Autodesk Inventor part; units mm, degrees
ref_plane "YZ Plane" through (0, 0, 0) normal (1, 0, 0) x (0, 1, 0)
ref_plane "XZ Plane" through (0, 0, 0) normal (0, 1, 0) x (-1, 0, 0)
ref_plane "XY Plane" through (0, 0, 0) normal (0, 0, 1) x (1, 0, 0)
sketch "Skizze1" plane through (0, 0, 0) normal (0, 0, 1) x (1, 0, 0)
  line L0 (-4.75, 4.75) -> (4.75, 4.75)
  line L1 (4.75, 4.75) -> (4.75, -4.75)
  line L2 (4.75, -4.75) -> (-4.75, -4.75)
  line L3 (-4.75, -4.75) -> (-4.75, 4.75)
  line L4 (-4.75, 4.75) -> (4.75, -4.75) construction
  line L5 (4.75, 4.75) -> (-4.75, -4.75) construction
  point P0 (0, 0)
  dimension "d0" = 9.5
  dimension "d1" = 9.5
extrude "Extrusion1" add sketch "Skizze1" along normal blind 3.5
sketch "Skizze2" plane through (0, 0, 3.5) normal (0, 0, 1) x (1, 0, 0)
  circle A0 centre (0, 0) radius 8.5
  dimension "d4" = 17
extrude "Extrusion2" add sketch "Skizze2" along normal blind 3
sketch "Skizze3" plane through (0, 0, 6.5) normal (0, 0, 1) x (1, 0, 0)
  circle A0 centre (0, 0) radius 7.4
  circle A1 centre (0, 0) radius 8.5
  dimension "d7" = 14.8
  dimension "d19" = 1.1
extrude "Extrusion3" add sketch "Skizze3" along normal blind 96 contours A0
sketch "Skizze4" plane through (0, 0, 102.5) normal (0, 0, 1) x (1, 0, 0)
  line L0 (-4.75, -4.75) -> (4.75, -4.75)
  line L1 (-4.75, 4.75) -> (4.75, 4.75)
  line L2 (4.75, 4.75) -> (4.75, -4.75)
  line L3 (4.75, -4.75) -> (-4.75, -4.75)
  line L4 (-4.75, -4.75) -> (-4.75, 4.75)
  line L5 (-4.75, 4.75) -> (4.75, -4.75) construction
  line L6 (4.75, 4.75) -> (-4.75, -4.75) construction
  point P0 (0, 0)
  dimension "d10" = 9.5
extrude "Extrusion4" add sketch "Skizze4" along normal blind 6
sketch "Skizze5" plane through (0, 0, 108.5) normal (0, 0, 1) x (1, 0, 0)
  circle A0 centre (0, 0) radius 2.25
  dimension "d13" = 4.5
extrude "Extrusion5" cut sketch "Skizze5" against normal blind 5
sketch "Skizze6" plane through (0, 0, 0) normal (0, 0, -1) x (-1, 0, 0)
  circle A0 centre (0, 0) radius 2.25
  dimension "d16" = 4.5
extrude "Extrusion6" cut sketch "Skizze6" against normal blind 5
properties part number "_3D-Druck"
Work out the finished part from the listing and answer in its coordinate system (mm). A direction names the side the tool comes from. Give positions to 0.01 mm unless a question says otherwise; leave off trailing zeros. Write each loop counter-clockwise with the first axis right and the second up, starting at its lowest first coordinate (ties: lowest second). Pieces come first, ordered by that corner, then holes.
(1) Flat-ended cylindrical pins translate along their axes: pin 1 Ø4 at (y, z) = (1.5, 2) entering from -X; pin 2 Ø1 at (x, y) = (1.5, 6) entering from -Z; pin 3 Ø3 at (x, z) = (2.5, 2.5) entering from -Y. Find the tip coordinate at first contact, or state that the pin passes through.
Final values:
pin 1: stops at x = -8.5
pin 2: stops at z = 3.5
pin 3: stops at y = -8.39
(2) The mould has two halves that part along X. Classify faces 5 (the cylindrical face through (0.29, 2.23, 2.46)), 6 (the flat face through (0, -6, 3.5)), 7 (the flat face through (4.75, 0, 2)): pulls with the +X half, pulls with the -X half, needs draft (parallel to the pull), parting line crosses it, or undercut.
Final values:
face 5: undercut
face 6: needs draft
face 7: pulls with the +X half
(3) The part is cut by section D-D on y = -6. Write down the section's boundary in (x, z).
Final values:
outline: (-6.02, 3.5) - (6.02, 3.5) - (6.02, 6.5) - (4.33, 6.5) - (4.33, 102.5) - (-4.33, 102.5) - (-4.33, 6.5) - (-6.02, 6.5) - close
(4) The part is cut by section A-A on x = 0. Write down the section's boundary in (y, z).
Final values:
outline: (-8.5, 3.5) - (-4.75, 3.5) - (-4.75, 0) - (-2.25, 0) - (-2.25, 5) - (2.25, 5) - (2.25, 0) - (4.75, 0) - (4.75, 3.5) - (8.5, 3.5) - (8.5, 6.5) - (7.4, 6.5) - (7.4, 102.5) - (4.75, 102.5) - (4.75, 108.5) - (2.25, 108.5) - (2.25, 103.5) - (-2.25, 103.5) - (-2.25, 108.5) - (-4.75, 108.5) - (-4.75, 102.5) - (-7.4, 102.5) - (-7.4, 6.5) - (-8.5, 6.5) - close
(5) Which of the six approach directions +Z, -Z, +X, -X, +Y, -Y give full straight-line access (tool end or side, diameter ignored) to faces 1 (the flat face through (0, -4.75, 105)), 2 (the flat face through (0, 0, 103.5)), 3 (the flat face through (0, 0, 5)), 4 (the flat face through (-4.75, 0, 105))?
Final values:
face 1: +Z, +X, -X, -Y
face 2: +Z
face 3: -Z
face 4: +Z, -X, +Y, -Y
(6) The part is cut by section C-C on z = 70. Write down the section's boundary in (x, y).
Final values:
outline: circle Ø14.8 at (0, 0)
(7) Straight lines are drawn through the part: line 1 (Y direction, x = 0, z = 105.55); line 2 (Z direction, x = 5.5, y = 2); line 3 (X direction, y = 0.25, z = 78.5). For each, find the intervals that lie inside material, in ascending order.
Final values:
line 1: y = -4.75 to -2.25, 2.25 to 4.75
line 2: z = 3.5 to 102.5
line 3: x = -7.4 to 7.4
